Study the drawing (mm; zero at the part's minimum x, y, z) and answer. A direction names the side the tool comes from. Give positions to 0.01 mm unless a question says otherwise; leave off trailing zeros. Loops run counter-clockwise (first coordinate to the right, second up) from the corner with the lowest first, then second, coordinate; pieces in that order, holes last. Notation, with made-up numbers: (43, 14.5) - (47, 14.5) arc R16 cw to (47, 44.5) - close; hole circle Ø5 at (60.5, 24.5). An arc over 180 degrees is marked (long way). Write item = value, one per line. Start each with the question number.
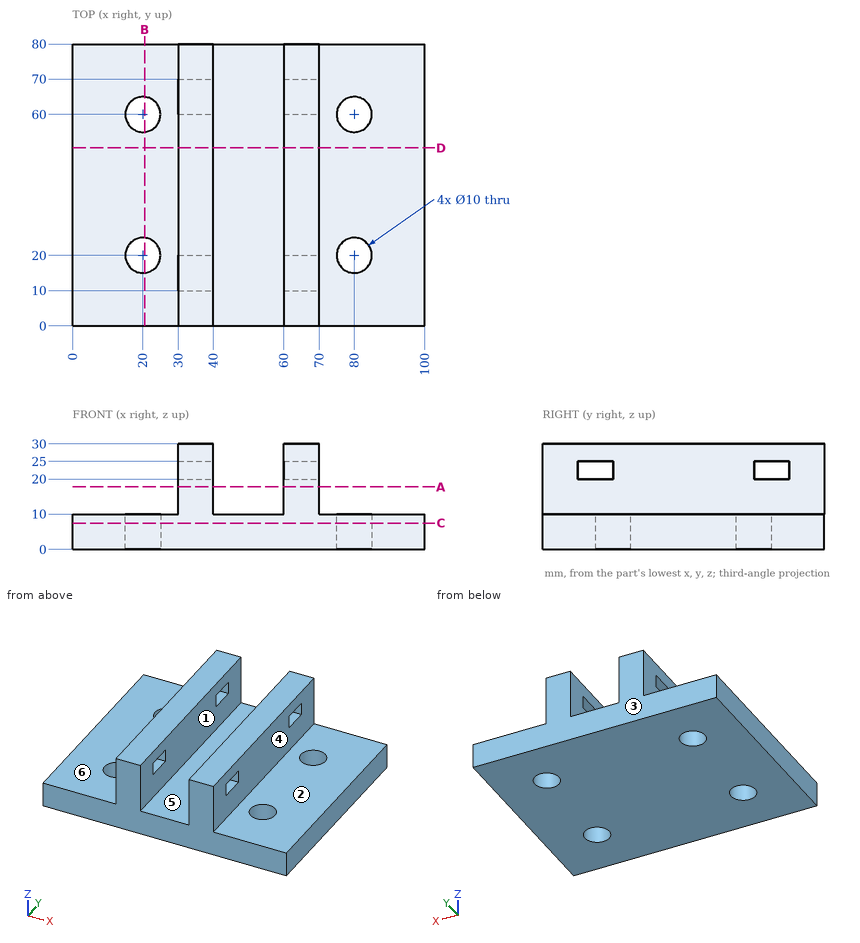
1. A tool of negligible diameter and unlimited length cuts with its end or side. For the marked faces 1, 2 and 3, from which of +Z, -Z, +X, -X, +Y, -Y can it reach the whole face along a straight path? Write none if from no direction.
2. Given P1, Ø1, axis at x = 29, y = 15, coming from the +Z side; P2, Ø10, axis at y = 48, z = 19, coming from the -X side; P3, Ø2, axis at y = 46.5, z = 25, coming from the +X side, each flat-ended and moving along its own axis, determine where each tip first touches the part or whether it passes through.
3. A cutting plane is placed at D-D on y = 50.5. Give the vertices of the cut face in (x, z), and give its area (3 significant figures).
4. A cutting plane is placed at C-C on z = 7.5. Give the vertices of the cut face in (x, y), and give its area (3 significant figures).
5. Consider line 1 along Y through (x, z) = (65, 21); line 2 along Y through (x, z) = (20, 5); line 3 along X through (y, z) = (27.5, 16). Determine where each line is inside the solid, lowest interval first. Write a range as [from, to].
6. A cutting plane is placed at A-A on z = 17.75. Give the vertices of the cut face in (x, y).
7. For a pull along X with two mould halves and no side action, classify the marked faces 4, 5 and 6 as released by +X, released by -X, zero draft, split by the parting line, or undercut.
8. A cutting plane is placed at B-B on x = 20.5. Give the vertices of the cut face in (y, z).
Reply:
q1.face_1 = +Z, +Y, -Y
q1.face_2 = +Z, +X, +Y, -Y
q1.face_3 = +Z, -Z, +X, -X, +Y
q2.P1 = 10
q2.P2 = 30
q2.P3 = 70
q3.outline = (0, 0) - (100, 0) - (100, 10) - (70, 10) - (70, 30) - (60, 30) - (60, 10) - (40, 10) - (40, 30) - (30, 30) - (30, 10) - (0, 10) - close
q3.area = 1,400 mm^2
q4.outline = (0, 0) - (100, 0) - (100, 80) - (0, 80) - close; hole circle Ø10 at (20, 20); hole circle Ø10 at (20, 60); hole circle Ø10 at (80, 20); hole circle Ø10 at (80, 60)
q4.area = 7,690 mm^2
q5.line_1 = [0, 10], [20, 60], [70, 80]
q5.line_2 = [0, 15], [25, 55], [65, 80]
q5.line_3 = [30, 40], [60, 70]
q6.outline = (30, 0) - (40, 0) - (40, 80) - (30, 80) - close; (60, 0) - (70, 0) - (70, 80) - (60, 80) - close
q7.face_4 = released by +X
q7.face_5 = undercut
q7.face_6 = zero draft
q8.outline = (0, 0) - (15.03, 0) - (15.03, 10) - (0, 10) - close; (24.97, 0) - (55.03, 0) - (55.03, 10) - (24.97, 10) - close; (64.97, 0) - (80, 0) - (80, 10) - (64.97, 10) - close
